```python
from build123d import *

# Parameters (mm, degrees)
F0_W     = 38.1
F0_H     = 38.1
F1_DEPTH = 38.1
F5_DEPTH = 38.1
F7_DEPTH = 38.1
F8_W     = 25.4
F8_H     = 7.62
F9_DEPTH = 38.1


with BuildPart() as f1:
    # F0 (on Front) → F1 (new body)
    with BuildSketch(Plane.XZ):
        with Locations((19.05, -19.05)):
            Rectangle(F0_W, F0_H)
    extrude(amount=F1_DEPTH)

    # F4 (on offset) → F5 (cut)
    with BuildSketch(Plane.YZ.offset(38.1)):
        Polygon((-31.75, -38.1), (-38.1, 0), (-38.1, -38.1), align=None)
        Polygon((-11.43, -28.104628), (-6.35, 0), (-31.75, 0), (-26.67, -28.104628), (-21.59, -9.525), (-16.51, -9.525), align=None)
        Polygon((-25.4, -38.1), (-12.7, -38.1), (-19.05, -22.225), align=None)
        Polygon((0, -32.925924), (0, 0), (-6.35, -38.1), (0, -38.1), align=None)
    extrude(amount=-F5_DEPTH, mode=Mode.SUBTRACT)

    # F6 (on offset) → F7 (cut)
    with BuildSketch(Plane.XZ.offset(38.1)):
        Polygon((6.35, 0), (0, 0), (0, -38.1), align=None)
        Polygon((25.4, 0), (12.7, 0), (19.05, -15.875), align=None)
        Polygon((11.43, -15.875), (6.35, -38.1), (31.75, -38.1), (26.67, -15.875), (21.59, -28.575), (16.51, -28.575), align=None)
        Polygon((38.1, 0), (31.75, 0), (38.1, -38.1), align=None)
    extrude(amount=-F7_DEPTH, mode=Mode.SUBTRACT)

    # F8 (on Top) → F9 (cut)
    with BuildSketch(Plane.XY):
        with Locations((25.4, -11.43)):
            Rectangle(F8_W, F8_H)
        with Locations((12.7, -26.67)):
            Rectangle(F8_W, F8_H)
    extrude(amount=-F9_DEPTH, mode=Mode.SUBTRACT)


solid = f1.part
```
Design review of the part built by this model. Coordinates are the model's own, in mm. A direction names the side the tool comes from. Give positions to 0.01 mm unless a question says otherwise; leave off trailing zeros. Loops run counter-clockwise (first coordinate to the right, second up) from the corner with the lowest first, then second, coordinate; pieces in that order, holes last. Notation, with made-up numbers: M 58.25,21.25 L 104.25,21.25 A23 cw 104.25,55.25 Z; hole C 15.5,9.25 d1. An arc over 180 degrees is marked long. Return JSON: item names as keys, results as strings. Group by question number.
Item 1: Insertion check: pin 1 Ø3 at (y, z) = (-29.5, -33.5) entering from -X; pin 2 Ø7.5 at (x, z) = (7, -28) entering from +Y; pin 3 Ø7.5 at (x, z) = (24.5, -24.5) entering from -Y. Each pin has a flat end and moves straight along its axis. Give the tip position at first contact, or say it passes through.
Item 2: Tool access review of faces 1 (the flat face through (13, -22.86, -19)), 2 (the flat face through (11.279, -22.234, -11.88)), 3 (the flat face through (28.68, -25.49, -24.67)), 4 (the flat face through (32.6, -17.1, -27.1)): name each direction out of +Z, -Z, +X, -X, +Y, -Y from which nothing blocks a thin tool from reaching the whole face with its end or side.
Item 3: We need section C-C (z = -25). Give the number of separate pieces and of enclosed holes in the cut face, and give its area (3 significant figures).
Item 4: Mouldability with a two-part tool opening along X and no side actions: class faces 5 (the flat face through (33.2, -22.2, -30.1)), 6 (the flat face through (19, -6, -28.575)), 7 (the flat face through (12.7, -8, -16)) as released by +X, released by -X, zero draft, split by the parting line, or undercut.
Item 5: For probe 1 along Y at (x, z) = (30, -23.5); probe 2 along X at (y, z) = (-21, -26); probe 3 along Y at (x, z) = (24, -17), list the stretches that pass through material, from the lowest coordinate up.
Item 6: We need section A-A (z = -3). Give the boundary of the cut face in (x, y), and give its area (3 significant figures).
Item 7: We need section D-D (z = -32.5). Give the boundary of the cut face in (x, y).
Output:
{
 "1": {"pin 1": "stops at x = 0.58", "pin 2": "stops at y = -4.04", "pin 3": "stops at y = -34.64"},
 "2": {"face 1": "+Z, -Z, -X", "face 2": "+Z, +X, -X", "face 3": "-Z, +Y, -Y", "face 4": "-Z, +X, -X"},
 "3": {"separate pieces": "12", "enclosed holes": "0", "area": "363 mm^2"},
 "4": {"face 5": "zero draft", "face 6": "undercut", "face 7": "released by +X"},
 "5": {"probe 1": "y = -34.18 to -27.5, -25.41 to -19.56, -18.54 to -15.24, -7.62 to -3.92", "probe 2": "x = 2.02 to 9.12, 15.48 to 22.62, 28.98 to 36.08", "probe 3": "y = -35.27 to -30.48, -22.86 to -15.24, -7.62 to -2.83"},
 "6": {"outline": "M 5.85,-37.6 L 13.9,-37.6 L 13.9,-31.21 L 5.85,-31.21 Z; M 5.85,-6.89 L 13.9,-6.89 L 13.9,-0.5 L 5.85,-0.5 Z; M 24.2,-37.6 L 32.25,-37.6 L 32.25,-31.21 L 24.2,-31.21 Z; M 24.2,-6.89 L 32.25,-6.89 L 32.25,-0.5 L 24.2,-0.5 Z", "area": "206 mm^2"},
 "7": {"outline": "M 0.93,-32.68 L 7.63,-32.68 L 7.63,-30.48 L 0.93,-30.48 Z; M 0.93,-14.94 L 7.63,-14.94 L 7.63,-5.42 L 0.93,-5.42 Z; M 30.47,-32.68 L 37.17,-32.68 L 37.17,-23.16 L 30.47,-23.16 Z; M 30.47,-7.62 L 37.17,-7.62 L 37.17,-5.42 L 30.47,-5.42 Z"}
}
